```python
from build123d import *

# Parameters (mm, degrees)
SKETCH1_W                      = 9.5
SKETCH1_H                      = 9.5
BOSS_EXTRUDE1_DEPTH            = 6
CUT_EXTRUDE1_DEPTH             = 3
M4_CLEARANCE_HOLE1_D           = 4.5
M4_CLEARANCE_HOLE1_CSINK_D     = 4.55
M4_CLEARANCE_HOLE1_CSINK_ANGLE = 90


with BuildPart() as part:
    # Sketch1 → Boss-Extrude1 (new body)
    with BuildSketch(Plane(origin=(0, 0, 0), x_dir=(1, 0, 0), z_dir=(0, 1, 0))):
        Rectangle(SKETCH1_W, SKETCH1_H)
    extrude(amount=BOSS_EXTRUDE1_DEPTH)

    # Sketch2 → Cut-Extrude1 (cut)
    with BuildSketch(Plane(origin=(0, 6, 0), x_dir=(1, 0, 0), z_dir=(0, 1, 0))):
        Polygon((0, -3.954849344), (3.425, -1.977424672), (3.425, 1.977424672), (0, 3.954849344), (-3.425, 1.977424672), (-3.425, -1.977424672), align=None)
    extrude(amount=-CUT_EXTRUDE1_DEPTH, mode=Mode.SUBTRACT)

    # M4 Clearance Hole1 (through all)
    with Locations(Plane(origin=(0, 3, 0), x_dir=(1, 0, 0), z_dir=(0, 1, 0))):
        with Locations((0, 0)):
            CounterSinkHole(M4_CLEARANCE_HOLE1_D / 2, M4_CLEARANCE_HOLE1_CSINK_D / 2, counter_sink_angle=M4_CLEARANCE_HOLE1_CSINK_ANGLE)


solid = part.part
```
Source: CAD feature listing. Evaluate the final solid. Frame: model axes, mm. A direction names the side the tool comes from. Give positions to 0.01 mm unless a question says otherwise; leave off trailing zeros. Loops run counter-clockwise (first coordinate to the right, second up) from the corner with the lowest first, then second, coordinate; pieces in that order, holes last. Notation, with made-up numbers: M -3,53 L 8,53 A8 cw 8,64 Z; hole C 82.5,65.5 d2. An arc over 180 degrees is marked long. Put each result on its own line as item: value.
Q1. Section D-D (y = 2.55). Return the cut outline in (x, z).
Response values:
outline: M -4.75,-4.75 L 4.75,-4.75 L 4.75,4.75 L -4.75,4.75 Z; hole C 0,0 d4.5
Q2. Pin query (flat end, axial travel): P1, Ø2, axis at x = 0, z = -1.5, coming from the +Y side. Return the tip coordinate at first contact, or that it passes through.
Response values:
P1: stops at y = 3
Q3. Section B-B (z = 0). Return the cut outline in (x, y) (3 decimals), and give its area (3 significant figures).
Response values:
outline: M -4.75,0 L -2.25,0 L -2.25,2.975 L -2.275,3 L -3.425,3 L -3.425,6 L -4.75,6 Z; M 2.25,0 L 4.75,0 L 4.75,6 L 3.425,6 L 3.425,3 L 2.275,3 L 2.25,2.975 Z
area: 22.9 mm²
Q4. Line query: probe 1 along Z at (x, y) = (0, 0.75); probe 2 along Y at (x, z) = (-1.25, 2); probe 3 along X at (y, z) = (3.95, 0.25) (3 decimals). Output: solid intervals per line, ascending. Write a range as [from, to].
Response values:
probe 1: z = [-4.75, -2.25], [2.25, 4.75]
probe 2: y = [0, 3]
probe 3: x = [-4.75, -3.425], [3.425, 4.75]
Q5. Mould query, pull axis Z, two halves, no side actions, for faces 1 (the flat face through (-4.75, 3, 0)), 2 (the flat face through (-1.69, 4.52, -2.98)), 3 (the flat face through (0, 3, -4.75)). Classes: released by +Z, released by -Z, zero draft, split by the parting line, or undercut.
Response values:
face 1: zero draft
face 2: undercut
face 3: released by -Z
Q6. Section A-A (y = 5). Return the cut outline in (x, z) (3 decimals).
Response values:
outline: M -4.75,-4.75 L 4.75,-4.75 L 4.75,4.75 L -4.75,4.75 Z; hole M -3.425,-1.977 L 0,-3.955 L 3.425,-1.977 L 3.425,1.977 L 0,3.955 L -3.425,1.977 Z
Q7. Section C-C (z = -3.25). Return the cut outline in (x, y), and give its area (3 significant figures).
Response values:
outline: M -4.75,0 L 4.75,0 L 4.75,6 L 1.22,6 L 1.22,3 L -1.22,3 L -1.22,6 L -4.75,6 Z
area: 49.7 mm²
Q8. Reachability of faces 4 (the flat face through (-2, 6, -3)), 5 (the flat face through (-2, 3, 2)) from +Z, -Z, +X, -X, +Y, -Y: full face, straight path, thin tool, end or side. Return the list, or none.
Response values:
face 4: +Z, -Z, +X, -X, +Y
face 5: +Y
